Answer from the drawing. Dimensions are ordinates in mm from the lowest x, y and z of the part. A direction names the side the tool comes from. Give positions to 0.01 mm unless a question says otherwise; leave off trailing zeros. Order: outer loops, then holes, each group sorted by start corner. A loop starts at its lowest first (then second) coordinate and runs counter-clockwise, first axis right, second up. Notation, with made-up numbers: (22.5, -12.5) -> (49.5, -12.5) arc R29 cw to (49.5, 12.5) -> close; hole circle Ø2 at (27.25, 32). An arc over 180 degrees is marked (long way). Write item = value, one per line. Start each with the question number.
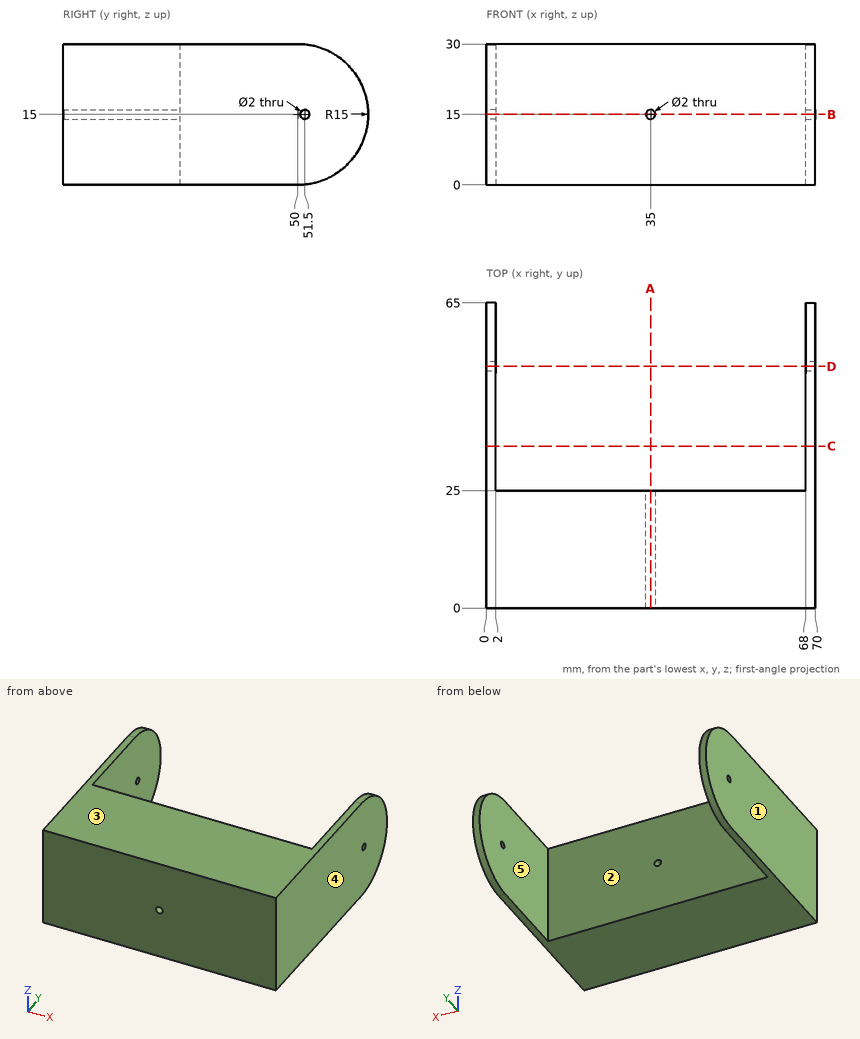
Item 1: Consider L1, parallel to X at y = 50.5, z = 28; L2, parallel to Z at x = 35, y = 9; L3, parallel to Y at x = 34.5, z = 2. Determine where each line is inside the solid, lowest interval first. Write a range as from..to.
Item 2: A cutting plane is placed at C-C, the plane y = 34.5. Write down the section's boundary in (x, z).
Item 3: Which of the six approach directions +Z, -Z, +X, -X, +Y, -Y give full straight-line access (tool end or side, diameter ignored) to the marked faces 4 and 5?
Item 4: The mould has two halves that part along X. Classify the marked faces 1, 2 and 3: +X half, -X half, draft (parallel to the pull), parting line (faces both ways), or undercut.
Item 5: Flat-ended cylindrical pins translate along their axes: pin 1 (1.2 mm diameter, centred on x = 35, z = 15, fed in from +Y); pin 2 (6 mm diameter, centred on x = 38.5, z = 24, fed in from +Y). Find the tip coordinate at first contact, or state that the pin passes through.
Item 6: A cutting plane is placed at A-A, the plane x = 35. Write down the section's boundary in (y, z), plus the area to 3 significant figures.
Item 7: A cutting plane is placed at D-D, the plane y = 51.5. Write down the section's boundary in (x, z).
Item 8: A cutting plane is placed at B-B, the plane z = 15. Write down the section's boundary in (x, y).
Check values:
q1.L1 = 0..2, 68..70
q1.L2 = 0..14, 16..30
q1.L3 = 0..25
q2.outline = (0, 0) -> (2, 0) -> (2, 30) -> (0, 30) -> close; (68, 0) -> (70, 0) -> (70, 30) -> (68, 30) -> close
q3.face_4 = +Z, -Z, +X, +Y, -Y
q3.face_5 = +Z, -Z, +Y
q4.face_1 = -X half
q4.face_2 = undercut
q4.face_3 = draft
q5.pin_1 = through
q5.pin_2 = 25
q6.outline = (0, 0) -> (25, 0) -> (25, 14) -> (0, 14) -> close; (0, 16) -> (25, 16) -> (25, 30) -> (0, 30) -> close
q6.area = 700 mm^2
q7.outline = (0, 0.08) -> (2, 0.08) -> (2, 14) -> (0, 14) -> close; (0, 16) -> (2, 16) -> (2, 29.92) -> (0, 29.92) -> close; (68, 0.08) -> (70, 0.08) -> (70, 14) -> (68, 14) -> close; (68, 16) -> (70, 16) -> (70, 29.92) -> (68, 29.92) -> close
q8.outline = (0, 0) -> (34, 0) -> (34, 25) -> (2, 25) -> (2, 50.5) -> (0, 50.5) -> close; (0, 52.5) -> (2, 52.5) -> (2, 65) -> (0, 65) -> close; (36, 0) -> (70, 0) -> (70, 50.5) -> (68, 50.5) -> (68, 25) -> (36, 25) -> close; (68, 52.5) -> (70, 52.5) -> (70, 65) -> (68, 65) -> close
